Design review of the part built by this model. Coordinates are the model's own, in mm. A direction names the side the tool comes from. Coordinates: 2 decimals unless noted, no trailing zeros. Write each loop counter-clockwise with the first axis right and the second up, starting at its lowest first coordinate (ties: lowest second). Pieces come first, ordered by that corner, then holes. Notation, with made-up numbers: (33, 47) -> (55, 47) arc R27 cw to (55, 67) -> close; hole circle Ø8 at (-36, 0.5). An arc over 180 degrees is marked (long way). Return JSON: item names as keys, results as strings. Group by question number.
from build123d import *

# Parameters (mm, degrees)
EXTRUDE_2_DEPTH  = 1
SKETCH_2_R       = 1.5
EXTRUDE_3_DEPTH  = 1
EXTRUDE_4_DEPTH  = 1
SKETCH_4_R       = 1.5
EXTRUDE_5_DEPTH  = 1
SKETCH_5_W       = 82
SKETCH_5_H       = 4
EXTRUDE_6_DEPTH  = 0.5
SKETCH_6_W       = 21
SKETCH_6_H       = 4
EXTRUDE_7_DEPTH  = 1
SKETCH_7_W       = 21
SKETCH_7_H       = 4
EXTRUDE_8_DEPTH  = 1
SKETCH_8_W       = 6
SKETCH_8_H       = 4
EXTRUDE_9_DEPTH  = 1
SKETCH_9_W       = 6
SKETCH_9_H       = 4
EXTRUDE_10_DEPTH = 1


with BuildPart() as part:
    # Sketch 1 → Extrude 2 (new body)
    with BuildSketch(Plane.XY.offset(19.5)):
        with BuildLine():
            Line((56.648774872, 85.153357287), (60.648774872, 85.153357287))
            Line((60.648774872, 85.153357287), (60.648774872, 46.653357287))
            ThreePointArc((60.648774872, 46.653357287), (61.148774872, 45.153357287), (60.648774872, 43.653357287))
            Line((60.648774872, 43.653357287), (60.648774872, -34.846642713))
            Line((60.648774872, -34.846642713), (56.648774872, -34.846642713))
            Line((56.648774872, -34.846642713), (56.648774872, 43.653357287))
            ThreePointArc((56.648774872, 43.653357287), (56.148774872, 45.153357287), (56.648774872, 46.653357287))
            Line((56.648774872, 46.653357287), (56.648774872, 85.153357287))
        make_face()
    extrude(amount=EXTRUDE_2_DEPTH)

    # Sketch 2 → Extrude 3 (add)
    with BuildSketch(Plane(origin=(0, 0, 19.5), x_dir=(-1, 0, 0), z_dir=(0, 0, -1))):
        with Locations((-58.648774872, 45.153357287)):
            Circle(SKETCH_2_R)
    extrude(amount=EXTRUDE_3_DEPTH)



with BuildPart() as body_2:
    # Sketch 3 → Extrude 4 (new body)
    with BuildSketch(Plane(origin=(0, 0, -19.5), x_dir=(-1, 0, 0), z_dir=(0, 0, -1))):
        with BuildLine():
            Line((17.351225128, 43.653357287), (17.351225128, -34.846642713))
            Line((17.351225128, -34.846642713), (21.351225128, -34.846642713))
            Line((21.351225128, -34.846642713), (21.351225128, 43.653357287))
            ThreePointArc((21.351225128, 43.653357287), (21.851225128, 45.153357287), (21.351225128, 46.653357287))
            Line((21.351225128, 46.653357287), (21.351225128, 85.153357287))
            Line((21.351225128, 85.153357287), (17.351225128, 85.153357287))
            Line((17.351225128, 85.153357287), (17.351225128, 46.653357287))
            ThreePointArc((17.351225128, 46.653357287), (16.851225128, 45.153357287), (17.351225128, 43.653357287))
        make_face()
    extrude(amount=EXTRUDE_4_DEPTH)

    # Sketch 4 → Extrude 5 (add)
    with BuildSketch(Plane.XY.offset(-19.5)):
        with Locations((-19.351225128, 45.153357287)):
            Circle(SKETCH_4_R)
    extrude(amount=EXTRUDE_5_DEPTH)


with BuildPart() as body_3:
    # Sketch 5 → Extrude 6 (new body, symmetric)
    with BuildSketch(Plane.XY):
        with Locations((19.648774872, 83.153357287)):
            Rectangle(SKETCH_5_W, SKETCH_5_H)
    extrude(amount=EXTRUDE_6_DEPTH, both=True)


with BuildPart() as part_1:
    add(part.part)

    add(body_3.part)  # Extrude 7 merges body 3
    # Sketch 6 → Extrude 7 (add)
    with BuildSketch(Plane(origin=(60.648774872, 0, 0), x_dir=(0, 0, -1), z_dir=(1, 0, 0))):
        with Locations((-10, 83.153357287)):
            Rectangle(SKETCH_6_W, SKETCH_6_H)
    extrude(amount=EXTRUDE_7_DEPTH)


    add(body_2.part)  # Extrude 8 merges body 2
    # Sketch 7 → Extrude 8 (add)
    with BuildSketch(Plane.ZY.offset(21.351225128)):
        with Locations((-10, 83.153357287)):
            Rectangle(SKETCH_7_W, SKETCH_7_H)
    extrude(amount=EXTRUDE_8_DEPTH)

    # Sketch 8 → Extrude 9 (add)
    with BuildSketch(Plane.XZ.offset(34.846642713)):
        with Locations((-20.351225128, -20)):
            Rectangle(SKETCH_8_W, SKETCH_8_H)
    extrude(amount=EXTRUDE_9_DEPTH)

    # Sketch 9 → Extrude 10 (add)
    with BuildSketch(Plane.XZ.offset(34.846642713)):
        with Locations((57.648774872, 20)):
            Rectangle(SKETCH_9_W, SKETCH_9_H)
    extrude(amount=EXTRUDE_10_DEPTH)


solid = part_1.part
Q1. For P1, Ø0.5, axis at y = 69, z = -20, coming from the -X side; P2, Ø1.5, axis at x = 58, y = 45.5, coming from the -Z side; P3, Ø3, axis at y = 83, z = -5.5, coming from the +X side, all flat-tipped, find the tip position at first contact; note any pin that passes through.
Q2. Wall thickness on L1, parallel to Z at x = 58.5, y = -7.5: over which ranges is the line inside the solid? List them lowest first.
Q3. For faces 4 (the flat face through (-20, -34.847, -19)), 5 (the cylindrical face through (-18.7, 43.8, -19)), 6 (the flat face through (-19, 24, -20.5)), 7 (the flat face through (58, 24, 20.5)), 8 (the flat face through (60.649, 4, 20)), list the 3-axis set-ups (+Z, -Z, +X, -X, +Y, -Y) from which the entire face can be reached by the end or side of a thin tool; tool diameter is ignored.
Q4. We need section C-C on z = -10. Write out the cut boundary in (x, y).
Q5. The part is to be moulded in two halves that separate along X. For faces 1 (the flat face through (58, -34.847, 21)), 2 (the flat face through (-22.351, 83, -10)), 3 (the cylindrical face through (58, 43.8, 19)), say which applies: +X half, -X half, draft (parallel to the pull), parting line (faces both ways), or undercut.
Q6. We need section B-B on x = 44.5. Write out the cut boundary in (y, z), plus the area to 3 significant figures.
Q7. We need section A-A on y = 27. Write out the cut boundary in (x, z), plus the area to 3 significant figures.
Findings below:
{
 "1": {"P1": "stops at x = -21.35", "P2": "stops at z = 18.5", "P3": "stops at x = -21.35"},
 "2": {"L1": "z = 19.5 to 20.5"},
 "3": {"face 4": "-X", "face 5": "+Z", "face 6": "-Z, +X, -X, +Y", "face 7": "+Z, +X, -X, +Y", "face 8": "+Z, -Z, +X, -Y"},
 "4": {"outline": "(-22.35, 81.15) -> (-21.35, 81.15) -> (-21.35, 85.15) -> (-22.35, 85.15) -> close"},
 "5": {"face 1": "draft", "face 2": "-X half", "face 3": "parting line"},
 "6": {"outline": "(81.15, -0.5) -> (85.15, -0.5) -> (85.15, 0.5) -> (81.15, 0.5) -> close", "area": "4.00 mm^2"},
 "7": {"outline": "(-21.35, -20.5) -> (-17.35, -20.5) -> (-17.35, -19.5) -> (-21.35, -19.5) -> close; (56.65, 19.5) -> (60.65, 19.5) -> (60.65, 20.5) -> (56.65, 20.5) -> close", "area": "8.00 mm^2"}
}
